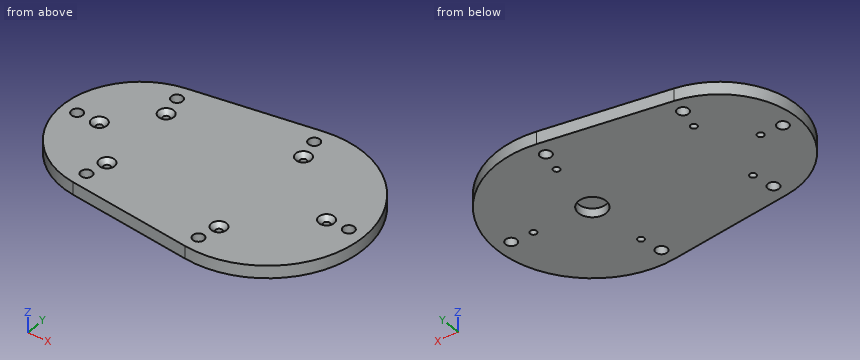
Autodesk Inventor part; units mm, degrees
ref_plane "YZ Plane" through (0, 0, 0) normal (1, 0, 0) x (0, 1, 0)
ref_plane "XZ Plane" through (0, 0, 0) normal (0, 1, 0) x (-1, 0, 0)
ref_plane "XY Plane" through (0, 0, 0) normal (0, 0, 1) x (1, 0, 0)
sketch "Sketch1" plane through (0, 0, 0) normal (0, 0, 1) x (1, 0, 0)
  arc A0 (-5.9149, 42.0864) -> (-5.9149, -42.0864) centre (0, 0) ccw
  arc A1 (92.2885, -55.888) -> (92.2885, 55.888) centre (100.143, 0) ccw
  line L0 (-42.5, 0) -> (156.5802, 0)
  line L1 (92.2885, 55.888) -> (-5.9149, 42.0864)
  line L2 (-5.9149, -42.0864) -> (92.2885, -55.888)
  line L3 (-3.1314, 22.281) -> (95.0719, 36.0826)
  arc A2 (95.0719, -36.0826) -> (95.0719, 36.0826) centre (100.143, 0) ccw
  line L4 (95.0719, -36.0826) -> (-3.1314, -22.281)
  arc A3 (-3.1314, 22.281) -> (-3.1314, -22.281) centre (0, 0) ccw
  circle A4 centre (100.143, 0) radius 11
  line L5 (89.505, -75.6933) -> (-8.6983, -61.8918)
  arc A5 (-8.6983, 61.8918) -> (-8.6983, -61.8918) centre (0, 0) ccw
  line L6 (-8.6983, 61.8918) -> (89.505, 75.6933)
  arc A6 (89.505, -75.6933) -> (89.505, 75.6933) centre (100.143, 0) ccw
  point P0 (146.5802, 0)
  point P1 (95.0719, 46.1809)
  point P2 (95.0719, -46.1809)
  point P3 (-32.5, 0)
  point P4 (-3.1314, 32.3793)
  point P5 (-3.1314, -32.3793)
  dimension "d0" = 85
  dimension "d1" = 100.143
  dimension "d2" = 8
  dimension "d3" = 20
  dimension "d4" = 10
  dimension "d5" = 10
  dimension "d6" = 10
  dimension "d7" = 10
  dimension "d8" = 10
  dimension "d9" = 10
  dimension "d22" = 22
  dimension "d26" = 20
extrude "Extrusion1" add sketch "Sketch1" along normal blind 10 contours L1 A1 L0 A2 L3 A3 A0 | L0 A3 L4 A2 A1 L2 A0 | A3 L3 A2 L0 A4 | L0 A4 A2 L4 A3 | L5 A5 L6 A6
sketch "Sketch4" plane through (0, 0, 10) normal (0, 0, 1) x (1, 0, 0)
  circle A0 centre (100.143, 0) radius 11.5
  point P0 (0, 0)
extrude "Extrusion4" add sketch "Sketch4" against normal blind 3
hole "Hole3" at (146.5802, 0, 0) at (95.0719, 46.1809, 0) at (95.0719, -46.1809, 0) at (-32.5, 0, 0) at (-3.1314, 32.3793, 0) at (-3.1314, -32.3793, 0) direction (0, 0, 1) diameter 5.2 end through all
sketch "Sketch8" plane through (0, 0, 0) normal (0, 0, -1) x (-1, 0, 0)
  circle A0 centre (6.9587, -49.5134) radius 4.5
  circle A1 centre (-164.0802, 0) radius 4.5
  circle A2 centre (6.9587, 49.5134) radius 4.5
  circle A3 centre (-91.2447, 63.315) radius 4.5
  circle A4 centre (-91.2447, -63.315) radius 4.5
  circle A5 centre (50, 0) radius 4.5
  line L0 (8.6983, -61.8918) -> (-89.505, -75.6933)
  arc A6 (8.6983, -61.8918) -> (8.6983, 61.8918) centre (0, 0) ccw
  line L1 (-89.505, 75.6933) -> (8.6983, 61.8918)
  arc A7 (-89.505, 75.6933) -> (-89.505, -75.6933) centre (-100.143, 0) ccw
  circle A8 centre (32.5, 0) radius 2.067
  circle A9 centre (3.1314, 32.3793) radius 2.067
  circle A10 centre (-95.0719, 46.1809) radius 2.067
  circle A11 centre (-146.5802, 0) radius 2.067
  arc A12 (-94.3761, 41.0339) -> (-94.3761, -41.0339) centre (-100.143, 0) ccw
  line L2 (3.8273, 27.2324) -> (-94.3761, 41.0339)
  arc A13 (3.8273, -27.2324) -> (3.8273, 27.2324) centre (0, 0) ccw
  line L3 (-94.3761, -41.0339) -> (3.8273, -27.2324)
  circle A14 centre (-95.0719, -46.1809) radius 2.067
  circle A15 centre (3.1314, -32.3793) radius 2.067
  circle A16 centre (3.1314, 32.3793) radius 2.6
  circle A17 centre (-95.0719, -46.1809) radius 2.6
  circle A18 centre (-146.5802, 0) radius 2.6
  circle A19 centre (-95.0719, 46.1809) radius 2.6
  circle A20 centre (32.5, 0) radius 2.6
  circle A21 centre (3.1314, -32.3793) radius 2.6
  line L4 (-89.505, 75.6933) -> (8.6983, 61.8918)
  arc A22 (-89.505, 75.6933) -> (-89.505, -75.6933) centre (-100.143, 0) ccw
  line L5 (8.6983, -61.8918) -> (-89.505, -75.6933)
  arc A23 (8.6983, -61.8918) -> (8.6983, 61.8918) centre (0, 0) ccw
hole "Hole6" at (164.0802, 0, 0) at (91.2447, -63.315, 0) at (-6.9587, -49.5134, 0) at (-50, 0, 0) at (-6.9587, 49.5134, 0) at (91.2447, 63.315, 0) direction (0, 0, 1) diameter 9 depth 40 tip angle 118
chamfer "Chamfer6" distance 3.5 angle 45 6 edges at (95.0719, 43.5809, 10) (146.5802, -2.6, 10) (95.0719, -48.7809, 10) (-3.1314, -34.9793, 10) (-32.5, -2.6, 10) (-3.1314, 29.7793, 10)
properties part number "onderkantBasegefreesd" material "Aluminum 6061"
Geometry: final body of the model. Coordinates: model frame, mm. Round coordinates to 2 decimals unless told otherwise and drop trailing zeros. Order: outer loops, then holes, each group sorted by start corner. A loop starts at its lowest first (then second) coordinate and runs counter-clockwise, first axis right, second up. Notation, with made-up numbers: (39, 49) - (96, 49) arc R24 cw to (96, 61) - close; hole circle Ø10 at (-25.75, -7). An arc over 180 degrees is marked (long way). Write each question's results on one line, items separated by ' | '.
Item 1: Section D-D, the plane x = 55.5. Return the cut outline in (y, z), and give its area (3 significant figures).
Completed:
outline: (-70.91, 0) - (70.91, 0) - (70.91, 10) - (-70.91, 10) - close | area: 1,420 mm^2
Item 2: Section B-B, the plane x = -32.5. Return the cut outline in (y, z), and give its area (3 significant figures).
Completed:
outline: (-53.39, 0) - (-2.6, 0) - (-2.6, 6.5) - (-6.1, 10) - (-53.39, 10) - close; (2.6, 0) - (53.39, 0) - (53.39, 10) - (6.1, 10) - (2.6, 6.5) - close | area: 1,000 mm^2
Item 3: Material intervals for line 1 along X through (y, z) = (0, 3.5); line 2 along Y through (x, z) = (-5.5, 6.25); line 3 along Y through (x, z) = (-8, 2.75), sorted ascending. Write a range as [from, to].
Completed:
line 1: [-62.5, -54.5], [-45.5, -35.1], [-29.9, 89.14], [111.14, 143.98], [149.18, 159.58], [168.58, 176.58] | line 2: [-62.34, -53.77], [-45.26, -33.45], [-31.31, 31.31], [33.45, 45.26], [53.77, 62.34] | line 3: [-61.99, -53.89], [-45.14, 45.14], [53.89, 61.99]
Item 4: Section C-C, the plane z = 2. State how many separate pieces and enclosed holes the cut face has, and give its area (3 significant figures).
Completed:
separate pieces: 1 | enclosed holes: 13 | area: 28,500 mm^2
Item 5: Section A-A, the plane y = 0. Return the cut outline in (x, z), and give its area (3 significant figures).
Completed:
outline: (-62.5, 0) - (-54.5, 0) - (-54.5, 10) - (-62.5, 10) - close; (-45.5, 0) - (-35.1, 0) - (-35.1, 6.5) - (-38.6, 10) - (-45.5, 10) - close; (-29.9, 0) - (89.14, 0) - (89.14, 7) - (111.14, 7) - (111.14, 0) - (143.98, 0) - (143.98, 6.5) - (140.48, 10) - (-26.4, 10) - (-29.9, 6.5) - close; (149.18, 0) - (159.58, 0) - (159.58, 10) - (152.68, 10) - (149.18, 6.5) - close; (168.58, 0) - (176.58, 0) - (176.58, 10) - (168.58, 10) - close | area: 1,930 mm^2
Item 6: First-contact query: pin 1 Ø8.5 at (x, y) = (-3.13, 32.38) entering from +Z; pin 2 Ø14.5 at (x, y) = (-50, 0) entering from +Z; pin 3 Ø2 at (x, z) = (-24.5, 2.5) entering from +Y; pin 4 Ø1 at (y, z) = (48, 4) entering from -X. Flat tips, straight axial feed; report the tip coordinate or a pass-through.
Completed:
pin 1: z = 8.15 | pin 2: z = 10 | pin 3: y = 57.91 | pin 4: x = -40.62
